Geometry check sheet. Reference: the model listing, model coordinates, mm. A direction names the side the tool comes from. Give positions to 0.01 mm unless a question says otherwise; leave off trailing zeros. Write each loop counter-clockwise with the first axis right and the second up, starting at its lowest first coordinate (ties: lowest second). Pieces come first, ordered by that corner, then holes. Notation, with made-up numbers: (45.25, 46.5) - (82.25, 46.5) arc R28 ccw to (82.25, 73.5) - close; hole circle Ø11 at (-6, 41.5). An arc over 180 degrees is marked (long way). One line per question, with ' | ' between items. Start each with the question number.
Q1. Release check for a two-part mould opening along X. For faces 4 (the face through (-0.1, 0, 21.3)), 5 (the face through (11.23, -2, 0)), 6 (the face through (-12.138, -2.418, 0.308)) record: +X half, -X half, draft (parallel to the pull), parting line (faces both ways), or undercut.
Q2. Section check A-A on x = 0. Record the boundary of the cut face in (y, z).
Q3. Section check B-B on z = -12. Record the boundary of the cut face in (x, y).
Q4. Gauge pin test, flat ends, axial feed: P1, Ø8, axis at x = -7, y = 12, coming from the +Z side; P2, Ø10, axis at x = -9, y = 9, coming from the -Z side; P3, Ø4, axis at y = 10, z = -1, coming from the -X side. Record the tip position at first contact, or that the pin passes through.
Q5. Thickness scan on L1, parallel to Z at x = 8.25, y = 11.5; L2, parallel to X at y = 4, z = 9.5; L3, parallel to Y at x = -0.75, z = 16.5. Record the ranges inside material, lowest first. Write a range as [from, to].
Q6. Set-up check for faces 1 (the face through (0, -2, 20.73)), 2 (the face through (-12.25, 7, 0)), 3 (the face through (12.25, 7, 0)): record each of +Z, -Z, +X, -X, +Y, -Y from which the full face is reachable in a straight line by a thin tool's end or side.
Q7. Section check C-C on y = 9.5. Record the boundary of the cut face in (x, z).
Autodesk Inventor part; units mm, degrees
ref_plane "YZ Plane" through (0, 0, 0) normal (1, 0, 0) x (0, 1, 0)
ref_plane "XZ Plane" through (0, 0, 0) normal (0, 1, 0) x (-1, 0, 0)
ref_plane "XY Plane" through (0, 0, 0) normal (0, 0, 1) x (1, 0, 0)
sketch "Sketch1" plane through (0, 0, 0) normal (0, 1, 0) x (-1, 0, 0)
  line L0 (-12.25, 21) -> (12.25, 21)
  line L1 (12.25, 21) -> (12.25, -21)
  line L2 (12.25, -21) -> (-12.25, -21)
  line L3 (-12.25, -21) -> (-12.25, 21)
  line L4 (-12.25, 21) -> (12.25, -21) construction
  line L5 (12.25, 21) -> (-12.25, -21) construction
  point P0 (0, 0)
  dimension "d0" = 24.5
  dimension "d1" = 42
extrude "Extrusion1" add sketch "Sketch1" along normal blind 14
sketch "Sketch2" plane through (0, 0, 0) normal (0, -1, 0) x (1, 0, 0)
  line L0 (12.5, -22) -> (-12.5, -22)
  line L1 (-12.5, -22) -> (-12.5, 22)
  line L2 (-12.5, 22) -> (12.5, 22)
  line L3 (12.5, 22) -> (12.5, -22)
  line L4 (12.5, -22) -> (-12.5, 22) construction
  line L5 (-12.5, -22) -> (12.5, 22) construction
  point P0 (0, 0)
  dimension "d4" = 25
  dimension "d5" = 44
extrude "Extrusion2" add sketch "Sketch2" along normal blind 2.8
fillet "Fillet1" radius 1.27 4 edges at (0, -2.8, 22) (12.5, -2.8, 0) (0, -2.8, -22) (-12.5, -2.8, 0)
sketch "Sketch3" plane through (0, -2.8, 0) normal (0, -1, 0) x (1, 0, 0)
  line L0 (-11.23, -20.73) -> (-11.23, 20.73)
  line L1 (11.23, -20.73) -> (-11.23, -20.73)
  line L2 (-11.23, -20.73) -> (-11.23, 20.73)
  line L3 (-11.23, 20.73) -> (11.23, 20.73)
  line L4 (11.23, 20.73) -> (11.23, -20.73)
  line L5 (11.23, -20.73) -> (-11.23, 20.73) construction
  line L6 (-11.23, -20.73) -> (11.23, 20.73) construction
  point P0 (0, 0)
extrude "Extrusion3" cut sketch "Sketch3" against normal blind 1.27
properties part number "BatteryVoltage"
Working result:
1) face 4: draft | face 5: undercut | face 6: -X half
2) outline: (-2.8, -20.73) arc R1.27 ccw to (-1.53, -22) - (0, -22) - (0, -21) - (14, -21) - (14, 21) - (0, 21) - (0, 22) - (-1.53, 22) arc R1.27 ccw to (-2.8, 20.73) - (-1.53, 20.73) - (-1.53, -20.73) - close
3) outline: (-12.5, -1.53) arc R1.27 ccw to (-11.23, -2.8) - (-11.23, -1.53) - (11.23, -1.53) - (11.23, -2.8) arc R1.27 ccw to (12.5, -1.53) - (12.5, 0) - (12.25, 0) - (12.25, 14) - (-12.25, 14) - (-12.25, 0) - (-12.5, 0) - close
4) P1: stops at z = 21 | P2: stops at z = -21 | P3: stops at x = -12.25
5) L1: z = [-21, 21] | L2: x = [-12.25, 12.25] | L3: y = [-1.53, 14]
6) face 1: -Y | face 2: +Z, -Z, -X, +Y | face 3: +Z, -Z, +X, +Y
7) outline: (-12.25, -21) - (12.25, -21) - (12.25, 21) - (-12.25, 21) - close
